Source: three-view drawing plus pictorial views. Frame: mm from the lowest corner of the part. A direction names the side the tool comes from. Round coordinates to 2 decimals unless told otherwise and drop trailing zeros. Loops run counter-clockwise (first coordinate to the right, second up) from the corner with the lowest first, then second, coordinate; pieces in that order, holes last. Notation, with made-up numbers: M -7.5,65 L 3.5,65 A28 ccw 3.5,104 Z; hole C -1,-7.75 d2. An arc over 180 degrees is marked long. Return JSON: item names as keys, results as strings. Group by question number.
1) Section B-B (z = 19.4). Output: boundary loops of the cut face in (x, y).
2) Contact query for flat-ended pins moving along their axis: P1, Ø2, axis at y = 38.5, z = 10.5, coming from the -X side; P2, Ø0.7, axis at x = 32, y = 18.5, coming from the +Z side. Output: stop coordinate, or through.
3) Section D-D (x = 6.9). Output: boundary loops of the cut face in (y, z).
4) Section A-A (x = 19.4). Output: boundary loops of the cut face in (y, z), plus the area to 3 significant figures.
5) Material intervals for line 1 (X direction, y = 18, z = 36) (1 decimal); line 2 (Y direction, x = 31.9, z = 38.15) (1 decimal); line 3 (Y direction, x = 34.5, z = 37), sorted ascending. Write a range as from..to.
6) Access query for the marked faces 1 and 2. Directions: +Z, -Z, +X, -X, +Y, -Y. A direction counts if a zero-diameter tool reaches every point of the face in a straight line with its end or side. Return the directions, or none.
7) Section C-C (y = 8). Output: boundary loops of the cut face in (x, z).
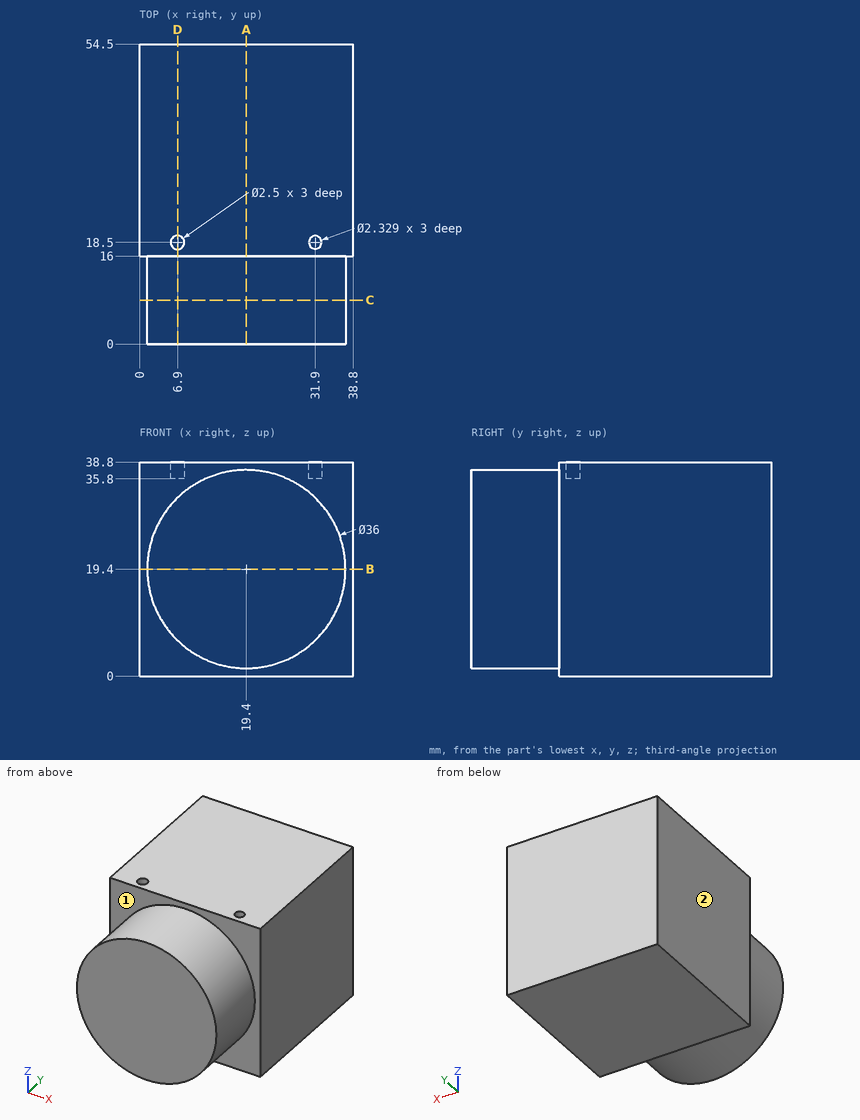
Returned:
{
 "1": {"outline": "M 0,16 L 1.4,16 L 1.4,0 L 37.4,0 L 37.4,16 L 38.8,16 L 38.8,54.5 L 0,54.5 Z"},
 "2": {"P1": "stops at x = 0", "P2": "stops at z = 35.8"},
 "3": {"outline": "M 0,6.45 L 16,6.45 L 16,0 L 54.5,0 L 54.5,38.8 L 19.75,38.8 L 19.75,35.8 L 17.25,35.8 L 17.25,38.8 L 16,38.8 L 16,32.35 L 0,32.35 Z"},
 "4": {"outline": "M 0,1.4 L 16,1.4 L 16,0 L 54.5,0 L 54.5,38.8 L 16,38.8 L 16,37.4 L 0,37.4 Z", "area": "2,070 mm^2"},
 "5": {"line 1": "x = 0..5.8, 8..30.8, 33..38.8", "line 2": "y = 16..17.3, 19.7..54.5", "line 3": "y = 16..54.5"},
 "6": {"face 1": "-Y", "face 2": "+Z, -Z, -X, +Y, -Y"},
 "7": {"outline": "C 19.4,19.4 d36"}
}
